```python
from build123d import *

# Parameters (mm, degrees)
SKETCH1_W           = 130.431067812
SKETCH1_H           = 127.071067812
SKETCH1_R           = 1.5
BOSS_EXTRUDE1_DEPTH = 2
CUT_EXTRUDE2_DEPTH  = 2
CUT_EXTRUDE3_DEPTH  = 2
SKETCH5_W           = 21.6
SKETCH5_H           = 31
CUT_EXTRUDE4_DEPTH  = 10
SKETCH6_R           = 1.5
CUT_EXTRUDE5_DEPTH  = 10
CUT_EXTRUDE6_DEPTH  = 10
CUT_EXTRUDE7_DEPTH  = 10


with BuildPart() as part:
    # Sketch1 → Boss-Extrude1 (new body)
    with BuildSketch(Plane(origin=(0, 0, 0), x_dir=(1, 0, 0), z_dir=(0, 1, 0))):
        with Locations((61.68, -60)):
            Rectangle(SKETCH1_W, SKETCH1_H)
        with Locations((0, -120)):
            Circle(SKETCH1_R, mode=Mode.SUBTRACT)
        with Locations((123.36, -120)):
            Circle(SKETCH1_R, mode=Mode.SUBTRACT)
        with Locations((123.36, 0)):
            Circle(SKETCH1_R, mode=Mode.SUBTRACT)
        Circle(SKETCH1_R, mode=Mode.SUBTRACT)
    extrude(amount=BOSS_EXTRUDE1_DEPTH)

    # Sketch3 → Cut-Extrude2 (cut)
    with BuildSketch(Plane(origin=(0, 2, 0), x_dir=(1, 0, 0), z_dir=(0, 1, 0))):
        Polygon((16.464466094, 3.535533906), (106.895533906, 3.535533906), (85.98014536, -39.812186932), (37.37985464, -39.812186932), align=None)
    extrude(amount=-CUT_EXTRUDE2_DEPTH, mode=Mode.SUBTRACT)

    # Sketch4 → Cut-Extrude3 (cut)
    with BuildSketch(Plane(origin=(0, 2, 0), x_dir=(1, 0, 0), z_dir=(0, 1, 0))):
        Polygon((85.98014536, -113.535533906), (37.37985464, -113.535533906), (16.464466094, -123.535533906), (106.895533906, -123.535533906), align=None)
    extrude(amount=-CUT_EXTRUDE3_DEPTH, mode=Mode.SUBTRACT)

    # Sketch5 → Cut-Extrude4 (cut)
    with BuildSketch(Plane(origin=(0, 2, 0), x_dir=(1, 0, 0), z_dir=(0, 1, 0))):
        with Locations((61.68, -88.035533906)):
            Rectangle(SKETCH5_W, SKETCH5_H)
    extrude(amount=-CUT_EXTRUDE4_DEPTH, mode=Mode.SUBTRACT)

    # Sketch6 → Cut-Extrude5 (cut)
    with BuildSketch(Plane(origin=(0, 2, 0), x_dir=(1, 0, 0), z_dir=(0, 1, 0))):
        with Locations((61.68, -64.535533906)):
            Circle(SKETCH6_R)
        with Locations((61.68, -49.535533906)):
            Circle(SKETCH6_R)
        with Locations((26.68, -57.035533906)):
            Circle(SKETCH6_R)
        with Locations((96.68, -57.035533906)):
            Circle(SKETCH6_R)
    extrude(amount=-CUT_EXTRUDE5_DEPTH, mode=Mode.SUBTRACT)

    # Sketch7 → Cut-Extrude6 (cut)
    with BuildSketch(Plane(origin=(0, 2, 0), x_dir=(1, 0, 0), z_dir=(0, 1, 0))):
        Polygon((31.68, -98.75817479), (36.68, -88.035533906), (31.68, -88.035533906), (26.68, -88.035533906), align=None)
        Polygon((36.68, -85.035533906), (26.68, -85.035533906), (31.68, -75.537485709), align=None)
        Polygon((86.68, -88.035533906), (91.68, -88.035533906), (96.68, -88.035533906), (91.68, -98.75817479), align=None)
        Polygon((86.68, -85.035533906), (91.68, -75.537485709), (96.68, -85.035533906), align=None)
    extrude(amount=-CUT_EXTRUDE6_DEPTH, mode=Mode.SUBTRACT)

    # Sketch8 → Cut-Extrude7 (cut)
    with BuildSketch(Plane(origin=(0, 2, 0), x_dir=(1, 0, 0), z_dir=(0, 1, 0))):
        Polygon((8.780452794, -60), (8.780452794, -43.363746638), (-3.535533906, -24.671327131), (-3.535533906, -88.786326042), (8.780452794, -74.953935606), align=None)
        Polygon((114.579547206, -43.363746638), (126.895533906, -24.671327131), (126.895533906, -88.786326042), (114.579547206, -74.953935606), (114.579547206, -60), align=None)
    extrude(amount=-CUT_EXTRUDE7_DEPTH, mode=Mode.SUBTRACT)


solid = part.part
```
Can you work these out from the model? Positions are in its coordinate system, mm. A direction names the side the tool comes from. Round coordinates to 2 decimals unless told otherwise and drop trailing zeros. Order: outer loops, then holes, each group sorted by start corner. A loop starts at its lowest first (then second) coordinate and runs counter-clockwise, first axis right, second up. Notation, with made-up numbers: (29, 9) -> (58, 9) arc R7 cw to (58, 21) -> close; hole circle Ø8 at (65, -31). An arc over 180 degrees is marked (long way). Return JSON: item names as keys, results as strings. Group by question number.
1. Which directions (+Z, -Z, +X, -X, +Y, -Y) give clear straight access to the entire face, cutting with the end or side of a thin tool? Please do faces 5 (the face through (120.824, 1.014, 81.967)), 6 (the face through (34.145, 1.014, 93.472)), 7 (the face through (2.536, 1.014, 81.967)), 8 (the face through (27.069, 1.014, 118.466)).
2. I need wall thicknesses on line 1 (Z direction, x = 61.68, y = 0.95); line 2 (X direction, y = 1.35, z = 77); line 3 (X direction, y = 1.8, z = 77.5). Which ranges of each line are inside material? Lowest first, please. Write a range as [from, to].
3. If we section it at C-C, the plane x = 123.36: Write out the boundary of the cut face in (y, z).
4. If we section it at B-B, the plane z = 101: Write out the boundary of the cut face in (x, y), then the cut area to 3 significant figures.
5. We'd pull the mould along Z, two halves only. Please class faces 1 (the face through (61, 0, 59)), 2 (the face through (97.372, 1.014, 58.366)), 3 (the face through (96.584, 1.014, 118.606)), 4 (the face through (60.49, 1.01, 50.45)): released by +Z, released by -Z, zero draft, split by the parting line, or undercut.
6. If we section it at D-D, the plane z = 60.5: Write out the boundary of the cut face in (x, y).
7. Will these pins go through, and if not, where does the flat tip stop? pin 1 (1 mm diameter, centred on x = 64, y = 1.5, fed in from -Z); pin 2 (5 mm diameter, centred on x = 123.36, z = 120, fed in from -Y); pin 3 (1 mm diameter, centred on x = 31, y = 1, fed in from +Z); pin 4 (0.6 mm diameter, centred on x = 93.5, y = 1.5, fed in from -Z).
8. If we section it at A-A, the plane x = 56: Write out the boundary of the cut face in (y, z).
Output values:
{
 "1": {"face 5": "+X, +Y, -Y", "face 6": "+Y, -Y", "face 7": "-X, +Y, -Y", "face 8": "+Z, +Y, -Y"},
 "2": {"line 1": "[39.81, 48.04], [51.04, 63.04], [66.04, 72.54], [103.54, 113.54]", "line 2": "[6.96, 30.91], [32.45, 50.88], [72.48, 90.91], [92.45, 116.4]", "line 3": "[6.51, 30.65], [32.71, 50.88], [72.48, 90.65], [92.71, 116.85]"},
 "3": {"outline": "(0, -3.54) -> (2, -3.54) -> (2, -1.5) -> (0, -1.5) -> close; (0, 1.5) -> (2, 1.5) -> (2, 30.04) -> (0, 30.04) -> close; (0, 84.82) -> (2, 84.82) -> (2, 118.5) -> (0, 118.5) -> close; (0, 121.5) -> (2, 121.5) -> (2, 123.54) -> (0, 123.54) -> close"},
 "4": {"outline": "(-3.54, 0) -> (50.88, 0) -> (50.88, 2) -> (-3.54, 2) -> close; (72.48, 0) -> (126.9, 0) -> (126.9, 2) -> (72.48, 2) -> close", "area": "218 mm²"},
 "5": {"face 1": "zero draft", "face 2": "undercut", "face 3": "released by +Z", "face 4": "undercut"},
 "6": {"outline": "(8.78, 0) -> (114.58, 0) -> (114.58, 2) -> (8.78, 2) -> close"},
 "7": {"pin 1": "z = 39.81", "pin 2": "y = 0", "pin 3": "z = 116.82", "pin 4": "z = 23.61"},
 "8": {"outline": "(0, 39.81) -> (2, 39.81) -> (2, 72.54) -> (0, 72.54) -> close; (0, 103.54) -> (2, 103.54) -> (2, 113.54) -> (0, 113.54) -> close"}
}
